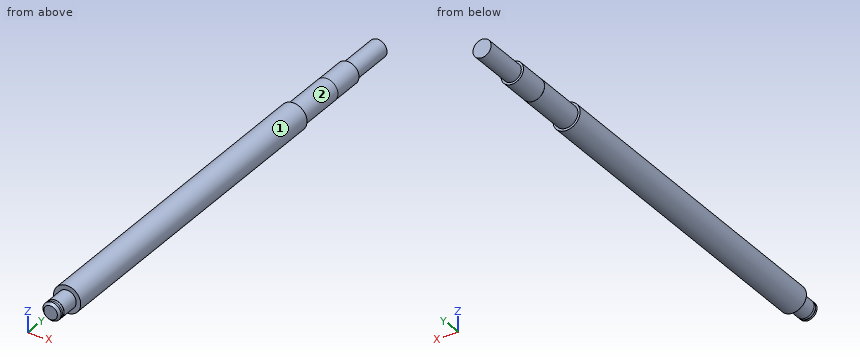
```python
from build123d import *

# Parameters (mm, degrees)
F0_R      = 6
F1_DEPTH  = 150
F2_R      = 5
F3_DEPTH  = 22
F4_R      = 4.95
F5_DEPTH  = 14
F6_R      = 4
F7_DEPTH  = 20
F8_R      = 4
F9_DEPTH  = 8
F10_R     = 3.9
F11_DEPTH = 1.15
F12_R     = 4
F13_DEPTH = 1.85
F14_SIZE  = 1


with BuildPart() as f1:
    # F0 (on Front) → F1 (new body)
    with BuildSketch(Plane.XZ):
        Circle(F0_R)
    extrude(amount=F1_DEPTH)

    # F2 (on face) → F3 (join)
    with BuildSketch(Plane(origin=(0, 0, 0), x_dir=(-1, 0, 0), z_dir=(0, 1, 0))):
        Circle(F2_R)
    extrude(amount=F3_DEPTH)

    # F4 (on face) → F5 (join)
    with BuildSketch(Plane(origin=(0, 22, 0), x_dir=(-1, 0, 0), z_dir=(0, 1, 0))):
        Circle(F4_R)
    extrude(amount=F5_DEPTH)

    # F6 (on face) → F7 (join)
    with BuildSketch(Plane(origin=(0, 36, 0), x_dir=(-1, 0, 0), z_dir=(0, 1, 0))):
        Circle(F6_R)
    extrude(amount=F7_DEPTH)

    # F8 (on face) → F9 (join)
    with BuildSketch(Plane.XZ.offset(150)):
        Circle(F8_R)
    extrude(amount=F9_DEPTH)

    # F10 (on face) → F11 (join)
    with BuildSketch(Plane.XZ.offset(158)):
        Circle(F10_R)
    extrude(amount=F11_DEPTH)

    # F12 (on face) → F13 (join)
    with BuildSketch(Plane.XZ.offset(159.15)):
        Circle(F12_R)
    extrude(amount=F13_DEPTH)

    # F14
    f14_edges = [f1.edges().sort_by_distance(p)[0] for p in [
        (-4, -161, 0),
    ]]
    chamfer(f14_edges, length=F14_SIZE)


solid = f1.part
```
CAD build for the part. Positions are in the model's coordinates, mm. Face numbers are marked on the shaded views. A direction names the side the tool comes from. Give positions to 0.01 mm unless a question says otherwise; leave off trailing zeros. Order: outer loops, then holes, each group sorted by start corner. A loop starts at its lowest first (then second) coordinate and runs counter-clockwise, first axis right, second up.
(1) Saw through at C-C, the plane y = -64. Give the cut face in (x, z), then the cut area to 3 significant figures.
(2) Flat gauge pin, fed straight in: pin 1 (6 mm diameter, centred on y = 11, z = -2.5, fed in from -X). Where does the tip first touch, or does it go through?
(3) Drill centre lines: L1, parallel to X at y = -140, z = 0.5; L2, parallel to Y at x = 4.75, z = -3. Where is each one in solid material? Low to high.
(4) Tool access for the marked faces 1 and 2: list every direction of +Z, -Z, +X, -X, +Y, -Y with a clear straight run to the whole face (end or side of a thin tool).
Results found:
1. outline: circle Ø12 at (0, 0)
1. area: 113 mm2
2. pin 1: stops at x = -5
3. L1: x = -5.98 to 5.98
3. L2: y = -150 to 0
4. face 1: +Y, -Y
4. face 2: +Y
